Check sheet for the drawn part. Datum: minimum x, y, z corner. Units: mm. A direction names the side the tool comes from. Round coordinates to 2 decimals unless told otherwise and drop trailing zeros. Order: outer loops, then holes, each group sorted by start corner. A loop starts at its lowest first (then second) coordinate and runs counter-clockwise, first axis right, second up.
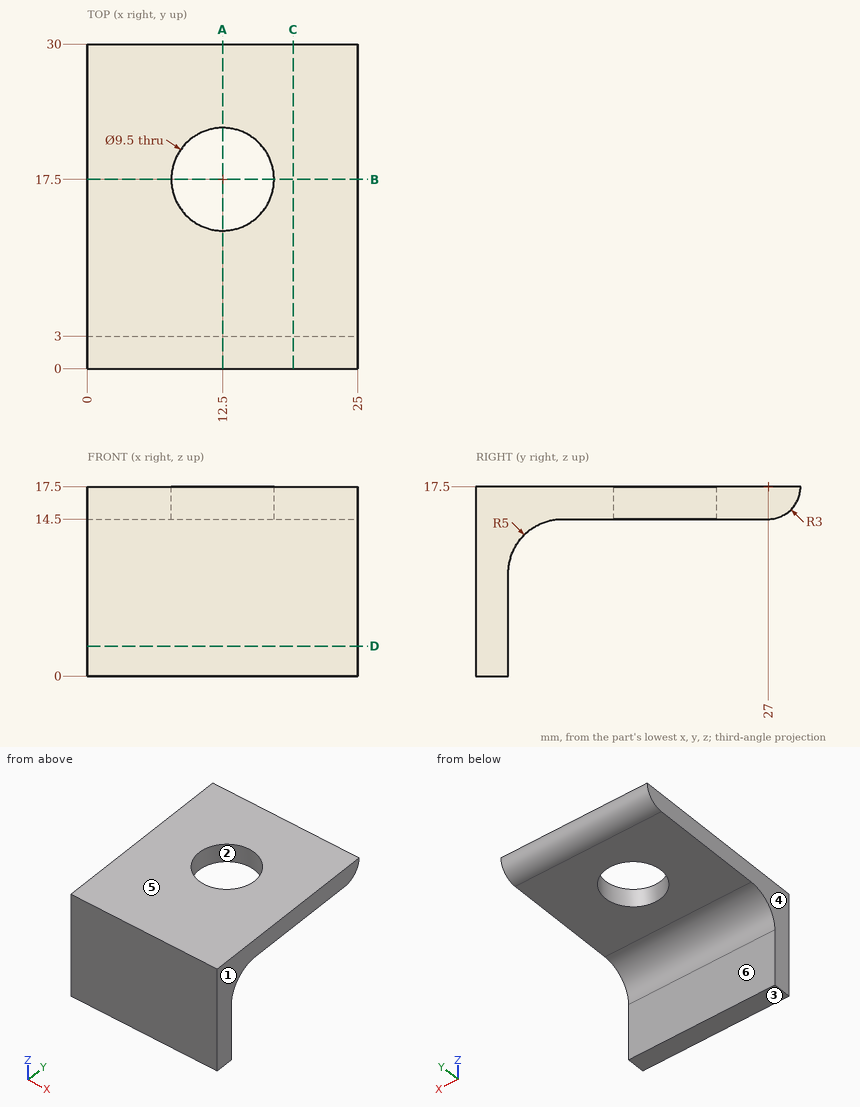
(1) Sectioned sample at D-D, the plane z = 2.75. Record the cut outline in (x, y).
Returned:
outline: (0, 0) - (25, 0) - (25, 3) - (0, 3) - close
(2) Sectioned sample at C-C, the plane x = 19. Record the cut outline in (y, z).
Returned:
outline: (0, 0) - (3, 0) - (3, 9.5) arc R5 cw to (8, 14.5) - (27, 14.5) arc R3 ccw to (30, 17.5) - (0, 17.5) - close
(3) Draft check along X on the marked faces 1, 2, 3 and 4. Enter one of: released by +X, released by -X, zero draft, split by the parting line, or undercut.
Returned:
face 1: released by +X
face 2: undercut
face 3: zero draft
face 4: released by -X
(4) Material ranges on line 1 (Z direction, x = 19.75, y = 16.75); line 2 (Y direction, x = 12.5, z = 16.5); line 3 (Y direction, x = 12.5, z = 15.35), recorded low to high.
Returned:
line 1: z = 14.5 to 17.5
line 2: y = 0 to 12.75, 22.25 to 29.83
line 3: y = 0 to 12.75, 22.25 to 29.09
(5) Set-up check for the marked faces 5 and 6: record each of +Z, -Z, +X, -X, +Y, -Y from which the full face is reachable in a straight line by a thin tool's end or side.
Returned:
face 5: +Z, +X, -X, +Y, -Y
face 6: -Z, +X, -X, +Y
(6) Sectioned sample at B-B, the plane y = 17.5. Record the cut outline in (x, z), and give its area (3 significant figures).
Returned:
outline: (0, 14.5) - (7.75, 14.5) - (7.75, 17.5) - (0, 17.5) - close; (17.25, 14.5) - (25, 14.5) - (25, 17.5) - (17.25, 17.5) - close
area: 46.5 mm2
(7) Depth check by flat-ended pin: P1, Ø15, axis at x = 8.5, y = 19.5, coming from the -Z side; P2, Ø1, axis at x = 11, z = 2.5, coming from the +Y side; P3, Ø10.5, axis at x = 12.5, z = 5.5, coming from the +Y side. Enter the tip coordinate at first touch or a pass-through.
Returned:
P1: stops at z = 14.5
P2: stops at y = 3
P3: stops at y = 3.16
(8) Sectioned sample at A-A, the plane x = 12.5. Record the cut outline in (y, z).
Returned:
outline: (0, 0) - (3, 0) - (3, 9.5) arc R5 cw to (8, 14.5) - (12.75, 14.5) - (12.75, 17.5) - (0, 17.5) - close; (22.25, 14.5) - (27, 14.5) arc R3 ccw to (30, 17.5) - (22.25, 17.5) - close
